Check sheet for the modelled part. Datum: model origin and axes. Units: mm. Round coordinates to 2 decimals unless told otherwise and drop trailing zeros. Order: outer loops, then holes, each group sorted by start corner. A loop starts at its lowest first (then second) coordinate and runs counter-clockwise, first axis right, second up. Notation, with made-up numbers: (62.25, 6.25) -> (85.25, 6.25) arc R15 cw to (85.25, 18.25) -> close; hole circle Ø11 at (-38, 35). An arc over 180 degrees is marked (long way). Answer in a Markdown table with one row per item. Add a question column.
1. Sectioned sample at A-A, the plane x = -1837.5. Record the boundary of the cut face in (y, z).
2. Material ranges on L1, parallel to X at y = -217.5, z = 14; L2, parallel to Y at x = -1304, z = 11; L3, parallel to Y at x = -1972, z = 13.5, recorded low to high. Write a range as from..to.
3. Sectioned sample at C-C, the plane z = 19.5. Record the boundary of the cut face in (x, y), then the cut area to 3 significant figures.
4. Depth check by flat-ended pin: P1, Ø10, axis at x = -1932.5, y = -211.5, coming from the +Z side; P2, Ø12.5, axis at y = -486.5, z = 16.5, coming from the +X side; P3, Ø20, axis at y = -1551, z = 17, coming from the -X side. Enter the tip coordinate at first touch or a pass-through.
5. Sectioned sample at B-B, the plane y = -374.5. Record the boundary of the cut face in (x, z), then the cut area to 3 significant figures.
```python
from build123d import *

# Parameters (mm, degrees)
F1_DEPTH = 30
F0_W     = 20
F0_H     = 30
F0_W_2   = 1020
F2_DEPTH = 35
F0_W_3   = 700
F0_H_2   = 70
F3_DEPTH = 25


with BuildPart() as f1:
    # F0 (on Top) → F1 (new body)
    with BuildSketch(Plane.XY):
        Polygon((-1947.5297451019, -160.4416549206), (-1877.5297451019, -160.4416549206), (-1177.5297451019, -160.4416549206), (-1107.5297451019, -160.4416549206), (-1067.5297451019, -160.4416549206), (-1017.5297451019, -110.4416549206), (-1017.5297451019, -80.4416549206), (-2037.5297451019, -80.4416549206), (-2037.5297451019, -110.4416549206), (-1987.5297451019, -160.4416549206), align=None)
    extrude(amount=F1_DEPTH)

    # F0 (on Top) → F2 (join)
    with BuildSketch(Plane.XY):
        with Locations((-2047.5297451019, -65.4416549206)):
            Rectangle(F0_W, F0_H)
        with Locations((-1527.5297451019, -65.4416549206)):
            Rectangle(F0_W_2, F0_H)
        with Locations((-1007.5297451019, -65.4416549206)):
            Rectangle(F0_W, F0_H)
    extrude(amount=F2_DEPTH)

    # F0 (on Top) → F3 (join)
    with BuildSketch(Plane.XY):
        Polygon((-1877.5297451019, -1460.4416549206), (-1877.5297451019, -160.4416549206), (-1947.5297451019, -160.4416549206), (-1947.5297451019, -1595.4416549206), (-1912.5297451019, -1595.4416549206), (-1877.5297451019, -1560.4416549206), (-1877.5297451019, -1530.4416549206), align=None)
        with Locations((-1527.5297451019, -1495.4416549206)):
            Rectangle(F0_W_3, F0_H_2)
        Polygon((-1107.5297451019, -160.4416549206), (-1177.5297451019, -160.4416549206), (-1177.5297451019, -1460.4416549206), (-1177.5297451019, -1530.4416549206), (-1177.5297451019, -1560.4416549206), (-1142.5297451019, -1595.4416549206), (-1107.5297451019, -1595.4416549206), align=None)
    extrude(amount=F3_DEPTH)


solid = f1.part
```
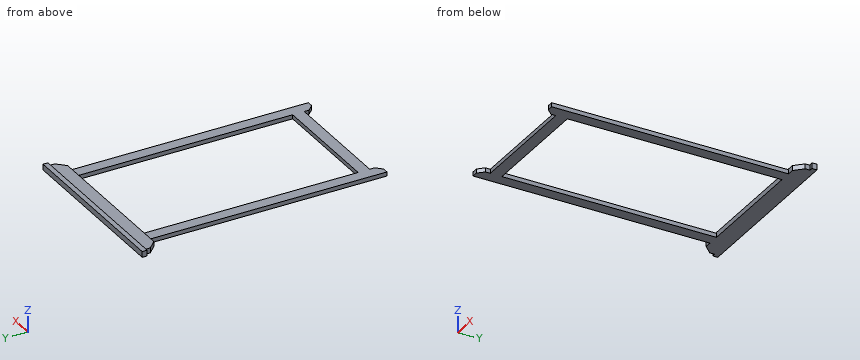
Answer key:
| question | item | result |
|---|---|---|
| 1 | outline | (-1530.44, 0) -> (-1460.44, 0) -> (-1460.44, 25) -> (-1530.44, 25) -> close; (-160.44, 0) -> (-50.44, 0) -> (-50.44, 35) -> (-80.44, 35) -> (-80.44, 30) -> (-160.44, 30) -> close |
| 2 | L1 | x = -1947.53..-1877.53, -1177.53..-1107.53 |
| 2 | L2 | y = -1530.44..-1460.44, -160.44..-50.44 |
| 2 | L3 | y = -160.44..-50.44 |
| 3 | outline | (-2057.53, -80.44) -> (-2037.53, -80.44) -> (-2037.53, -110.44) -> (-1987.53, -160.44) -> (-1947.53, -160.44) -> (-1947.53, -1595.44) -> (-1912.53, -1595.44) -> (-1877.53, -1560.44) -> (-1877.53, -1530.44) -> (-1177.53, -1530.44) -> (-1177.53, -1560.44) -> (-1142.53, -1595.44) -> (-1107.53, -1595.44) -> (-1107.53, -160.44) -> (-1067.53, -160.44) -> (-1017.53, -110.44) -> (-1017.53, -80.44) -> (-997.53, -80.44) -> (-997.53, -50.44) -> (-2057.53, -50.44) -> close; hole (-1877.53, -1460.44) -> (-1177.53, -1460.44) -> (-1177.53, -160.44) -> (-1877.53, -160.44) -> close |
| 3 | area | 360,000 mm² |
| 4 | P1 | stops at z = 25 |
| 4 | P2 | stops at x = -1107.53 |
| 4 | P3 | stops at x = -1947.53 |
| 5 | outline | (-1947.53, 0) -> (-1877.53, 0) -> (-1877.53, 25) -> (-1947.53, 25) -> close; (-1177.53, 0) -> (-1107.53, 0) -> (-1107.53, 25) -> (-1177.53, 25) -> close |
| 5 | area | 3,500 mm² |
